Source: CAD feature listing. Evaluate the final solid. Frame: model axes, mm. Face numbers are marked on the shaded views. A direction names the side the tool comes from. Round coordinates to 2 decimals unless told otherwise and drop trailing zeros. Order: outer loops, then holes, each group sorted by start corner. A loop starts at its lowest first (then second) coordinate and runs counter-clockwise, first axis right, second up. Notation, with made-up numbers: (-4, 83.25) -> (11, 83.25) arc R15 ccw to (11, 90.25) -> close; hole circle Ø4 at (86, 5.25). An arc over 180 degrees is marked (long way). One line per item, written item: value. Start each with the question number.
1) Mould query, pull axis Z, two halves, no side actions, for the marked faces 3, 4, 5 and 6. Classes: pulls with the +Z half, pulls with the -Z half, needs draft (parallel to the pull), parting line crosses it, or undercut.
2) Section A-A (y = -4.5). Return the cut outline in (x, z) (3 decimals).
3) Pin query (flat end, axial travel): P1, Ø1, axis at x = -1.5, y = 3, coming from the +Z side; P2, Ø3, axis at x = -2, z = -55, coming from the +Y side; P3, Ø3, axis at x = 2.5, y = 10, coming from the +Z side. Return the tip coordinate at first contact, or that it passes through.
4) Reachability of the marked faces 1 and 2 from +Z, -Z, +X, -X, +Y, -Y: full face, straight path, thin tool, end or side. Return the list, or none.
5) Ray query, L1, parallel to Y at x = 2.25, z = -2.5; L2, parallel to Z at x = 1.5, y = -1; L3, parallel to X at y = 1.75, z = -3 (3 decimals). Return the intervals inside material, ascending.
6) Section B-B (x = 3.75). Return the cut outline in (y, z), and give its area (3 significant figures).
7) Section C-C (z = -54.5). Return the cut outline in (x, y) (3 decimals), and give its area (3 significant figures).
```python
from build123d import *

# Parameters (mm, degrees)
BOSS_EXTRUDE1_DEPTH = 6.35
SKETCH3_R           = 1.9558
BOSS_EXTRUDE3_DEPTH = 10.16
SKETCH4_R           = 1.9558
BOSS_EXTRUDE4_DEPTH = 10.16
CUT_EXTRUDE1_DEPTH  = 66.761600688
FILLET2_R           = 0.635
CHAMFER4_SIZE       = 0.508


with BuildPart() as part:
    # Sketch1 → Boss-Extrude1 (new body)
    with BuildSketch(Plane(origin=(0, 0, 0), x_dir=(1, 0, 0), z_dir=(0, 1, 0))):
        with BuildLine():
            Line((-4.445, 0), (-4.445, 59.055))
            ThreePointArc((-4.445, 59.055), (0, 63.5), (4.445, 59.055))
            Line((4.445, 59.055), (4.445, 0))
            ThreePointArc((4.445, 0), (0, -4.445), (-4.445, 0))
        make_face()
    extrude(amount=BOSS_EXTRUDE1_DEPTH)

    # Sketch3 → Boss-Extrude3 (add)
    with BuildSketch(Plane(origin=(0, 6.35, 0), x_dir=(1, 0, 0), z_dir=(0, 1, 0))):
        with Locations(Location((0, 0, 0), (0, 0, 270))):
            Circle(SKETCH3_R)
    extrude(amount=BOSS_EXTRUDE3_DEPTH)

    # Sketch4 → Boss-Extrude4 (add)
    with BuildSketch(Plane.XZ):
        with Locations(Location((0, -59.055, 0), (0, 0, 90))):
            Circle(SKETCH4_R)
    extrude(amount=BOSS_EXTRUDE4_DEPTH)

    # Sketch5 → Cut-Extrude1 (cut, through all)
    with BuildSketch(Plane(origin=(0, 6.35, 0), x_dir=(1, 0, 0), z_dir=(0, 1, 0))):
        with BuildLine():
            Line((-4.445, 59.055), (-4.445, 0))
            ThreePointArc((-4.445, 0), (0.015635542, 29.5275), (-4.445, 59.055))
        make_face()
    extrude(amount=-CUT_EXTRUDE1_DEPTH, mode=Mode.SUBTRACT)

    # Fillet2
    fillet2_edges = [part.edges().sort_by_distance(p)[0] for p in [
        (0, 6.35, -1.9558),
        (0, 0, -61.0108),
    ]]
    fillet(fillet2_edges, radius=FILLET2_R)

    # Chamfer4
    chamfer4_edges = [part.edges().sort_by_distance(p)[0] for p in [
        (0, 16.51, -1.9558),
        (0, -10.16, -61.0108),
    ]]
    chamfer(chamfer4_edges, length=CHAMFER4_SIZE)


solid = part.part
```
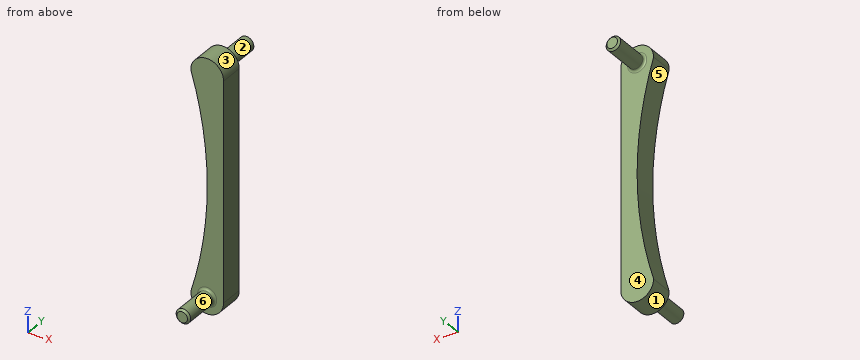
Findings:
1. face 3: pulls with the +Z half
1. face 4: needs draft
1. face 5: undercut
1. face 6: parting line crosses it
2. outline: circle Ø3.912 at (0, -59.055)
3. P1: z = 4.33
3. P2: y = 6.35
3. P3: z = 1.68
4. face 1: -Z, +Y, -Y
4. face 2: +Y
5. L1: 0 to 6.35
5. L2: -60.31 to -57.8
5. L3: -3.569 to 4.445
6. outline: (0, -61.44) -> (6.35, -61.44) -> (6.35, 2.39) -> (0, 2.39) -> close
6. area: 405 mm2
7. outline: (-3.154, 0) -> (4.445, 0) -> (4.445, 6.35) -> (-3.154, 6.35) -> close
7. area: 48.3 mm2
